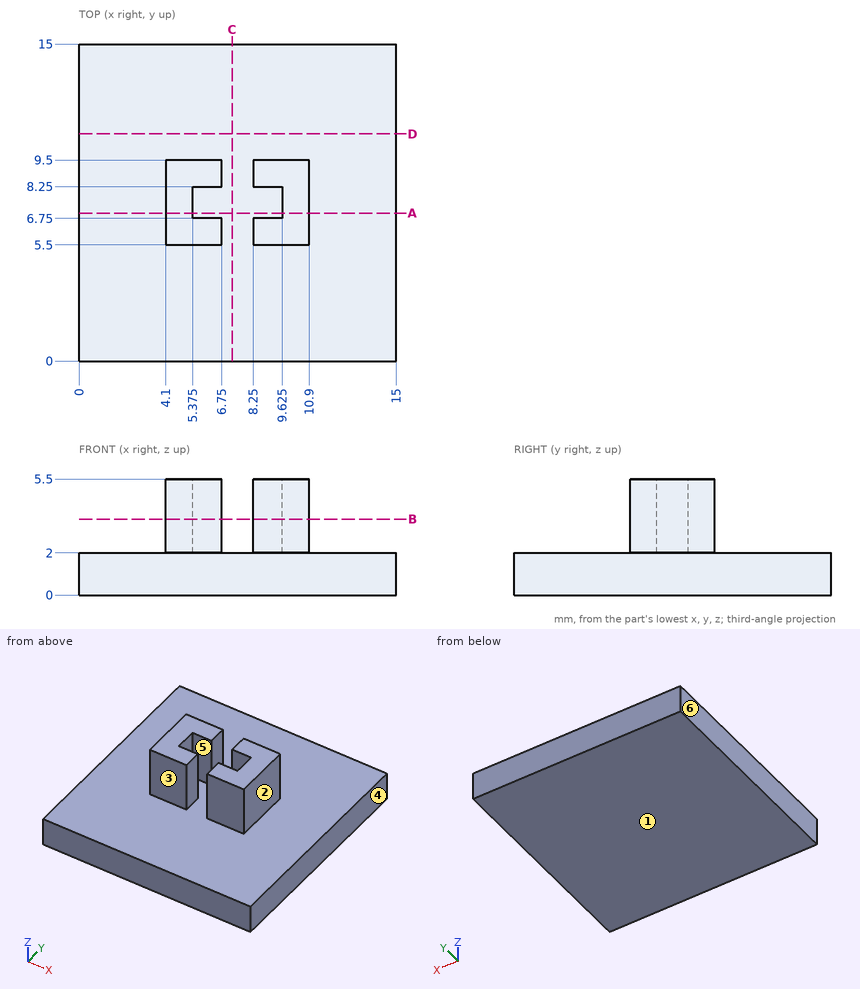
Answer from the drawing. Dimensions are ordinates in mm from the lowest x, y and z of the part. A direction names the side the tool comes from. Round coordinates to 2 decimals unless told otherwise and drop trailing zeros. Loops run counter-clockwise (first coordinate to the right, second up) from the corner with the lowest first, then second, coordinate; pieces in that order, holes last.
(1) The mould has two halves that part along X. Classify the marked faces 4, 5 and 6: pulls with the +X half, pulls with the -X half, needs draft (parallel to the pull), parting line crosses it, or undercut.
Computed values:
face 4: pulls with the +X half
face 5: undercut
face 6: pulls with the -X half
(2) Find the intervals of material crossed by L1, parallel to Y at x = 9.25, z = 2.15; L2, parallel to X at y = 6.5, z = 4.4; L3, parallel to X at y = 7, z = 4.4 (3 decimals), in increasing order.
Computed values:
L1: y = 5.5 to 6.75, 8.25 to 9.5
L2: x = 4.1 to 6.75, 8.25 to 10.9
L3: x = 4.1 to 5.375, 9.625 to 10.9
(3) Each of these flat-tipped pins is pushed along its axis until it touches: P1, Ø0.8, axis at x = 5, z = 3.5, coming from the +Y side; P2, Ø3, axis at x = 10, z = 4.5, coming from the -Y side; P3, Ø1.2, axis at y = 7.5, z = 3, coming from the +X side. Where does it stop, or does it pass through?
Computed values:
P1: stops at y = 9.5
P2: stops at y = 5.5
P3: stops at x = 10.9
(4) The part is cut by section C-C, the plane x = 7.25. Give the vertices of the cut face in (y, z), and give its area (3 significant figures).
Computed values:
outline: (0, 0) - (15, 0) - (15, 2) - (0, 2) - close
area: 30.0 mm2
(5) The part is cut by section A-A, the plane y = 7. Give the vertices of the cut face in (x, z) (3 decimals).
Computed values:
outline: (0, 0) - (15, 0) - (15, 2) - (10.9, 2) - (10.9, 5.5) - (9.625, 5.5) - (9.625, 2) - (5.375, 2) - (5.375, 5.5) - (4.1, 5.5) - (4.1, 2) - (0, 2) - close
(6) For the marked faces 1, 2 and 3, determine the directions among +Z, -Z, +X, -X, +Y, -Y from which every point of the face is accessible in a straight line to the end or side of a thin tool.
Computed values:
face 1: -Z, +X, -X, +Y, -Y
face 2: +Z, +X, +Y, -Y
face 3: +Z, +X, -X, -Y
(7) The part is cut by section B-B, the plane z = 3.6. Give the vertices of the cut face in (x, y) (3 decimals).
Computed values:
outline: (4.1, 5.5) - (6.75, 5.5) - (6.75, 6.75) - (5.375, 6.75) - (5.375, 8.25) - (6.75, 8.25) - (6.75, 9.5) - (4.1, 9.5) - close; (8.25, 5.5) - (10.9, 5.5) - (10.9, 9.5) - (8.25, 9.5) - (8.25, 8.25) - (9.625, 8.25) - (9.625, 6.75) - (8.25, 6.75) - close
